Here's the drawing with two shaded views (mm, measured from the low corner). I have some questions. A direction names the side the tool comes from. Coordinates: 2 decimals unless noted, no trailing zeros. Loops run counter-clockwise (first coordinate to the right, second up) from the corner with the lowest first, then second, coordinate; pieces in that order, holes last.
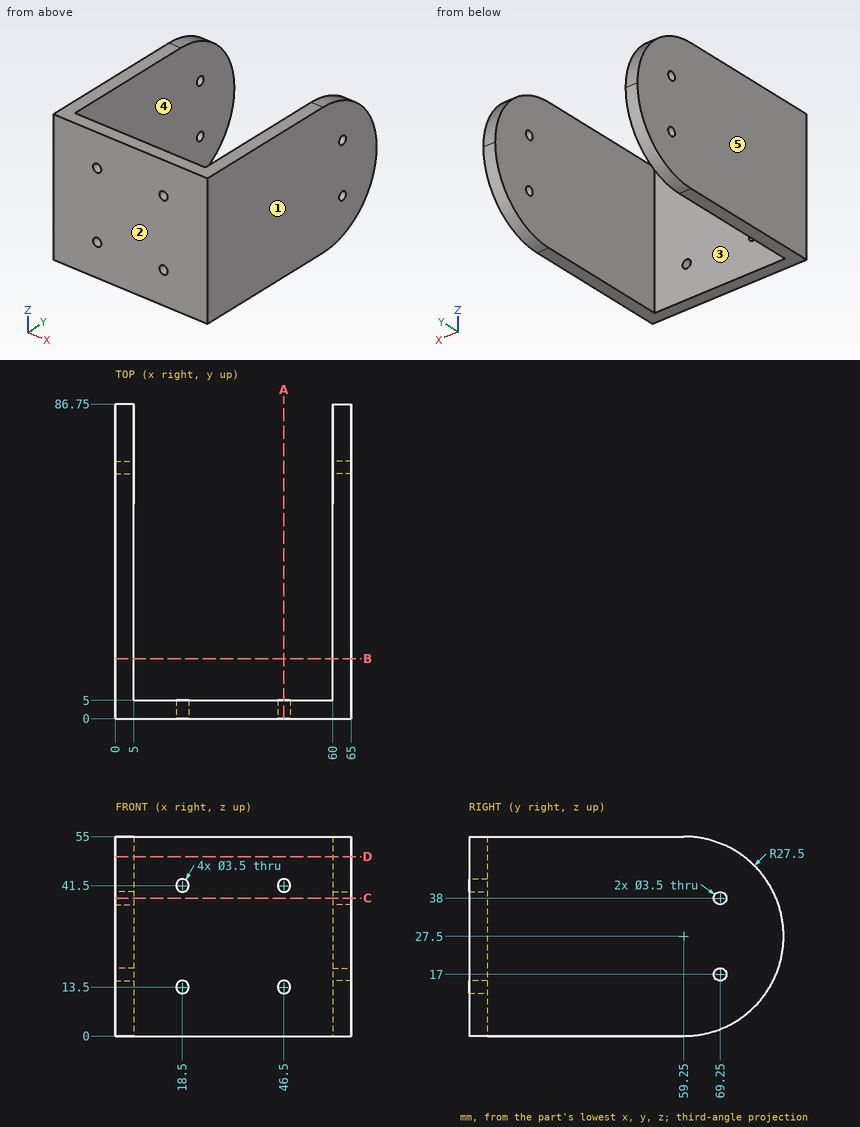
Q1. Suppose I cut it at B-B on y = 16.5. Write out the boundary of the cut face in (x, z), and give its area (3 significant figures).
Q2. We'd pull the mould along X, two halves only. Please class the marked faces 1, 2 and 3: pulls with the +X half, pulls with the -X half, needs draft (parallel to the pull), parting line crosses it, or undercut.
Q3. Suppose I cut it at A-A on x = 46.5. Write out the boundary of the cut face in (y, z), and give its area (3 significant figures).
Q4. For the marked faces 4 and 5, which set-ups out of +Z, -Z, +X, -X, +Y, -Y let a thin tool reach every point of the face, with its end or its side?
Q5. Suppose I cut it at C-C on z = 38. Write out the boundary of the cut face in (x, y).
Q6. Will this pin go through, and if not, where does the flat tip stop? P1, Ø10, axis at x = 39, z = 25, coming from the +Y side.
Q7. Please list where these lines run through material, in increasing order: probe 1 along X at (y, z) = (73.5, 17.5); probe 2 along X at (y, z) = (1.6, 41.5); probe 3 along Y at (x, z) = (10, 42.5).
Q8. Suppose I cut it at D-D on z = 49.5. Write out the boundary of the cut face in (x, y), and give its area (3 significant figures).
Check values:
1. outline: (0, 0) - (5, 0) - (5, 55) - (0, 55) - close; (60, 0) - (65, 0) - (65, 55) - (60, 55) - close
1. area: 550 mm2
2. face 1: pulls with the +X half
2. face 2: needs draft
2. face 3: undercut
3. outline: (0, 0) - (5, 0) - (5, 11.75) - (0, 11.75) - close; (0, 15.25) - (5, 15.25) - (5, 39.75) - (0, 39.75) - close; (0, 43.25) - (5, 43.25) - (5, 55) - (0, 55) - close
3. area: 240 mm2
4. face 4: +Z, -Z, +Y
4. face 5: +Z, -Z, -X, +Y, -Y
5. outline: (0, 0) - (65, 0) - (65, 67.5) - (60, 67.5) - (60, 5) - (5, 5) - (5, 67.5) - (0, 67.5) - close; (0, 71) - (5, 71) - (5, 84.67) - (0, 84.67) - close; (60, 71) - (65, 71) - (65, 84.67) - (60, 84.67) - close
6. P1: stops at y = 5
7. probe 1: x = 0 to 5, 60 to 65
7. probe 2: x = 0 to 16.75, 20.25 to 44.75, 48.25 to 65
7. probe 3: y = 0 to 5
8. outline: (0, 0) - (65, 0) - (65, 75.75) - (60, 75.75) - (60, 5) - (5, 5) - (5, 75.75) - (0, 75.75) - close
8. area: 1,030 mm2
